```python
from build123d import *

# Parameters (mm, degrees)
PLASTINA_DEPTH        = 3
OTVERSTIYA_DEPTH      = 62.362552644
OTVERSTIYA_DEPTH_BACK = 62.362552644
ESKIZ_OTVERSTIYA_R    = 1.65


with BuildPart() as part:
    # Eskiz_kontur → Plastina (new body)
    with BuildSketch(Plane.XY):
        with BuildLine():
            Line((17.26275, 53.34327), (10.40166, 21.0644))
            ThreePointArc((10.40166, 21.0644), (5.0644, 17.59834), (1.59834, 22.9356))
            Line((1.59834, 22.9356), (8.45942, 55.21447))
            ThreePointArc((8.45942, 55.21447), (13.796685, 58.680535), (17.26275, 53.34327))
        make_face()
    extrude(amount=PLASTINA_DEPTH)

    # Eskiz_otverstiya → Otverstiya (cut, two sides: drawn at the far end of the back side and taken through both)
    with BuildSketch(Plane.XY.offset(-OTVERSTIYA_DEPTH_BACK)):
        with Locations((6, 22)):
            Circle(ESKIZ_OTVERSTIYA_R)
        with Locations((12.86109, 54.27887)):
            Circle(ESKIZ_OTVERSTIYA_R)
    extrude(amount=OTVERSTIYA_DEPTH + OTVERSTIYA_DEPTH_BACK, mode=Mode.SUBTRACT)


solid = part.part
```
Input: part model. Units: mm. Frame: model coordinates. Coordinates: 2 decimals unless noted, no trailing zeros. Write each loop counter-clockwise with the first axis right and the second up, starting at its lowest first coordinate (ties: lowest second). Pieces come first, ordered by that corner, then holes. Notation, with made-up numbers: (74.25, 59) - (131.25, 59) arc R19 cw to (131.25, 94) - close; hole circle Ø2 at (19.5, 49.25). An arc over 180 degrees is marked (long way). Put each result on its own line as item: value. Start each with the question number.
1) Mould query, pull axis X, two halves, no side actions, for faces 1 (the face through (13.88, 37.43, 1.48)), 2 (the face through (13.622, 52.815, 1.479)), 3 (the face through (13.7, 58.7, 1.5)). Classes: pulls with the +X half, pulls with the -X half, needs draft (parallel to the pull), parting line crosses it, or undercut.
2) Cut plane D-D (y = 44.5). Return the cut outline in (x, z).
3) Cut plane B-B (z = 0.7). Return the cut outline in (x, y), plus the area to 3 significant figures.
4) Contact query for flat-ended pins moving along their axis: pin 1 (1 mm diameter, centred on x = 11, z = 0.5, fed in from +Y); pin 2 (1.5 mm diameter, centred on y = 33, z = 2, fed in from +X). Output: stop coordinate, or through.
5) Cut plane A-A (x = 5.5). Return the cut outline in (y, z).
6) Cut plane C-C (y = 22). Return the cut outline in (x, z), plus the area to 3 significant figures.
7) Ray query, L1, parallel to X at y = 20.5, z = 2.8; L2, parallel to X at y = 22, z = 0.75; L3, parallel to X at y = 36.5, z = 0.4. Return the intervals inside material, ascending.
Resolved:
1. face 1: pulls with the +X half
1. face 2: undercut
1. face 3: parting line crosses it
2. outline: (6.18, 0) - (15.38, 0) - (15.38, 3) - (6.18, 3) - close
3. outline: (1.6, 22.94) arc R4.5 ccw to (10.4, 21.06) - (17.26, 53.34) arc R4.5 ccw to (8.46, 55.21) - close; hole circle Ø3.3 at (6, 22); hole circle Ø3.3 at (12.86, 54.28)
3. area: 344 mm2
4. pin 1: stops at y = 58.57
4. pin 2: stops at x = 13.1
5. outline: (17.53, 0) - (20.43, 0) - (20.43, 3) - (17.53, 3) - close; (23.57, 0) - (41.29, 0) - (41.29, 3) - (23.57, 3) - close
6. outline: (1.5, 0) - (4.35, 0) - (4.35, 3) - (1.5, 3) - close; (7.65, 0) - (10.6, 0) - (10.6, 3) - (7.65, 3) - close
6. area: 17.4 mm2
7. L1: x = 1.76 to 5.31, 6.69 to 10.24
7. L2: x = 1.5 to 4.35, 7.65 to 10.6
7. L3: x = 4.48 to 13.68
